```python
from build123d import *

# Parameters (mm, degrees)
SALIENTE_EXTRUIR1_DEPTH = 5.9
SALIENTE_EXTRUIR2_DEPTH = 2.5
SALIENTE_EXTRUIR2_DRAFT = -10
VACIADO1_START          = -8.5
VACIADO1_DEPTH          = 17
VACIADO1_START_2        = -19.25
VACIADO1_2_DEPTH        = 38.5
SKETCH1_R               = 3.5
BOSS_EXTRUDE1_DEPTH     = 0.5
SKETCH2_R               = 2.65
SKETCH2_R_2             = 1.8
BOSS_EXTRUDE2_DEPTH     = 4
SKETCH3_R               = 0.55
CUT_EXTRUDE1_DEPTH      = 10


with BuildPart() as part:
    # Croquis1 → Saliente-Extruir1 (new body)
    with BuildSketch(Plane.XY):
        with BuildLine():
            Line((-20.25, 8.5), (-20.25, -8.5))
            ThreePointArc((-20.25, -8.5), (-19.957106781, -9.207106781), (-19.25, -9.5))
            Line((-19.25, -9.5), (19.25, -9.5))
            ThreePointArc((19.25, -9.5), (19.957106781, -9.207106781), (20.25, -8.5))
            Line((20.25, -8.5), (20.25, 8.5))
            ThreePointArc((20.25, 8.5), (19.957106781, 9.207106781), (19.25, 9.5))
            Line((19.25, 9.5), (-19.25, 9.5))
            ThreePointArc((-19.25, 9.5), (-19.957106781, 9.207106781), (-20.25, 8.5))
        make_face()
    extrude(amount=SALIENTE_EXTRUIR1_DEPTH)


with BuildPart() as saliente_extruir2_tool:
    # Croquis1<2> → Saliente-Extruir2 (with draft: the straight prism first)
    with BuildSketch(Plane.XY):
        with BuildLine():
            Line((-20.25, 8.5), (-20.25, -8.5))
            ThreePointArc((-20.25, -8.5), (-19.957106781, -9.207106781), (-19.25, -9.5))
            Line((-19.25, -9.5), (19.25, -9.5))
            ThreePointArc((19.25, -9.5), (19.957106781, -9.207106781), (20.25, -8.5))
            Line((20.25, -8.5), (20.25, 8.5))
            ThreePointArc((20.25, 8.5), (19.957106781, 9.207106781), (19.25, 9.5))
            Line((19.25, 9.5), (-19.25, 9.5))
            ThreePointArc((-19.25, 9.5), (-19.957106781, 9.207106781), (-20.25, 8.5))
        make_face()
    extrude(amount=-SALIENTE_EXTRUIR2_DEPTH)
    # Saliente-Extruir2: the draft: its side faces are tilted about the plane it starts from
    saliente_extruir2_sides = [saliente_extruir2_tool.faces().sort_by_distance(p)[0] for p in [
        (0, 9.5, -1.25),
        (-19.957106781, 9.207106781, -1.25),
        (-20.25, 0, -1.25),
        (-19.957106781, -9.207106781, -1.25),
        (0, -9.5, -1.25),
        (19.957106781, -9.207106781, -1.25),
        (20.25, 0, -1.25),
        (19.957106781, 9.207106781, -1.25),
    ]]
    draft(saliente_extruir2_sides, Plane.XY, SALIENTE_EXTRUIR2_DRAFT)


with BuildPart() as part_1:
    add(part.part)

    # Saliente-Extruir2: add saliente_extruir2_tool
    add(saliente_extruir2_tool.part)

    # Vaciado1: read off the stored shape, not the designer's step
    # Vaciado1 outline → Vaciado1 (cut)
    with BuildSketch(Plane(origin=(0, 0, 0), x_dir=(1, 0, 0), z_dir=(0, 1, 0)).offset(VACIADO1_START)):
        Polygon((-19.25, -0.087488664), (-19.25, -5.9), (19.25, -5.9), (19.25, -0.087488664), (18.970082917, 1.5), (-18.970082917, 1.5), align=None)
    extrude(amount=VACIADO1_DEPTH, mode=Mode.SUBTRACT)

    # Vaciado1 2 outline → Vaciado1 2 (add)
    with BuildSketch(Plane.YZ.offset(VACIADO1_START_2)):
        Polygon((8.5, 0.087488664), (8.220082917, -1.5), (8.5, -1.5), align=None)
        Polygon((-8.220082917, -1.5), (-8.5, 0.087488664), (-8.5, -1.5), align=None)
    extrude(amount=VACIADO1_2_DEPTH)

    # Sketch1 → Boss-Extrude1 (add)
    with BuildSketch(Plane(origin=(0, 0, -2.5), x_dir=(-1, 0, 0), z_dir=(0, 0, -1))):
        with Locations(Location((10.95, 0, 0), (0, 0, 180))):
            Circle(SKETCH1_R)
    extrude(amount=BOSS_EXTRUDE1_DEPTH)

    # Sketch2 → Boss-Extrude2 (add)
    with BuildSketch(Plane(origin=(0, 0, -3), x_dir=(-1, 0, 0), z_dir=(0, 0, -1))):
        with Locations((10.95, 0)):
            Circle(SKETCH2_R)
        with Locations((10.95, 0)):
            Circle(SKETCH2_R_2, mode=Mode.SUBTRACT)
    extrude(amount=BOSS_EXTRUDE2_DEPTH)

    # Sketch3 → Cut-Extrude1 (cut)
    with BuildSketch(Plane(origin=(0, 0, -2.5), x_dir=(-1, 0, 0), z_dir=(0, 0, -1))):
        with Locations((-18.309182548, -7.559182548)):
            Circle(SKETCH3_R)
        with Locations(Location((-18.309182548, 7.559182548, 0), (0, 0, 180))):
            Circle(SKETCH3_R)
    extrude(amount=-CUT_EXTRUDE1_DEPTH, mode=Mode.SUBTRACT)


solid = part_1.part
```
Source: CAD feature listing. Evaluate the final solid. Frame: model axes, mm. A direction names the side the tool comes from. Give positions to 0.01 mm unless a question says otherwise; leave off trailing zeros. Write each loop counter-clockwise with the first axis right and the second up, starting at its lowest first coordinate (ties: lowest second). Pieces come first, ordered by that corner, then holes.
1. Section query A-A (x = -10.95). Return the cut outline in (y, z), then the cut area to 3 significant figures.
2. Section query D-D (y = -6.5). Return the cut outline in (x, z).
3. Pull-direction query (Y, two-part tool) for faces 4 (the face through (19.965, 9.199, 2.909)), 5 (the face through (0, -8.5, 3)), 6 (the face through (-19.81, -9.05, -1.23)), 7 (the face through (20.033, -0.119, -1.233)); classes: +Y half, -Y half, draft (parallel to the pull), parting line (faces both ways), or undercut.
4. Material intervals for line 1 along Y through (x, z) = (8, 5.5); line 2 along Y through (x, z) = (-10.95, -4.05); line 3 along X through (y, z) = (2, 3), sorted ascending.
5. Section query C-C (z = -4). Return the cut outline in (x, y), then the cut area to 3 significant figures.
6. First-contact query: pin 1 (6 mm diameter, centred on x = 11.5, z = -5, fed in from -Y); pin 2 (1.5 mm diameter, centred on y = -6.5, z = -2.5, fed in from -X); pin 3 (4.5 mm diameter, centred on x = -10.95, y = 0, fed in from +Z); pin 4 (0.9 mm diameter, centred on x = 18.31, y = -7.56, fed in from +Z). Flat tips, straight axial feed; report the tip coordinate or a pass-through.
7. Section query B-B (y = 0). Return the cut outline in (x, z).
8. Access query for faces 1 (the face through (17.87, 7.89, -2.01)), 2 (the face through (-11, 0, -3)), 3 (the face through (-19.25, 0, 3)). Directions: +Z, -Z, +X, -X, +Y, -Y. A direction counts if a zero-diameter tool reaches every point of the face in a straight line with its end or side. Return the directions, or none.
Output values:
1. outline: (-9.5, 0) - (-9.06, -2.5) - (-3.5, -2.5) - (-3.5, -3) - (-2.65, -3) - (-2.65, -7) - (-1.8, -7) - (-1.8, -3) - (1.8, -3) - (1.8, -7) - (2.65, -7) - (2.65, -3) - (3.5, -3) - (3.5, -2.5) - (9.06, -2.5) - (9.5, 0) - (9.5, 5.9) - (8.5, 5.9) - (8.5, 0.09) - (8.22, -1.5) - (-8.22, -1.5) - (-8.5, 0.09) - (-8.5, 5.9) - (-9.5, 5.9) - close
1. area: 43.4 mm2
2. outline: (-20.25, 0) - (-19.81, -2.5) - (19.81, -2.5) - (20.25, 0) - (20.25, 5.9) - (19.25, 5.9) - (19.25, 0.09) - (18.97, -1.5) - (-18.97, -1.5) - (-19.25, 0.09) - (-19.25, 5.9) - (-20.25, 5.9) - close
3. face 4: +Y half
3. face 5: undercut
3. face 6: -Y half
3. face 7: draft
4. line 1: y = -9.5 to -8.5, 8.5 to 9.5
4. line 2: y = -2.65 to -1.8, 1.8 to 2.65
4. line 3: x = -20.25 to -19.25, 19.25 to 20.25
5. outline: circle Ø5.3 at (-10.95, 0); hole circle Ø3.6 at (-10.95, 0)
5. area: 11.9 mm2
6. pin 1: stops at y = -9.15
6. pin 2: stops at x = -19.94
6. pin 3: stops at z = -1.5
6. pin 4: passes through
7. outline: (-20.25, 0) - (-19.81, -2.5) - (-14.45, -2.5) - (-14.45, -3) - (-13.6, -3) - (-13.6, -7) - (-12.75, -7) - (-12.75, -3) - (-9.15, -3) - (-9.15, -7) - (-8.3, -7) - (-8.3, -3) - (-7.45, -3) - (-7.45, -2.5) - (19.81, -2.5) - (20.25, 0) - (20.25, 5.9) - (19.25, 5.9) - (19.25, 0.09) - (18.97, -1.5) - (-18.97, -1.5) - (-19.25, 0.09) - (-19.25, 5.9) - (-20.25, 5.9) - close
8. face 1: +Z, -Z
8. face 2: -Z
8. face 3: +Z
